Autodesk Inventor part; units mm, degrees
ref_plane "Work Plane1" through (-24, -152, 0) normal (0, -1, 0) x (1, 0, 0)
ref_plane "YZ Plane" through (0, 0, 0) normal (1, 0, 0) x (0, 1, 0)
ref_plane "XZ Plane" through (0, 0, 0) normal (0, 1, 0) x (-1, 0, 0)
sketch "Sketch1" plane through (0, 0, 0) normal (0, 0, 1) x (1, 0, 0)
  arc A0 (24, 0) -> (-24, 0) centre (0, 0) ccw
  line L0 (-24, 0) -> (-24, -152)
  line L1 (24, 0) -> (24, -152)
  dimension "d0" = 48
  dimension "d1" = 152
ref_plane "Work Plane1" through (-24, -152, 0) normal (0, -1, 0) x (1, 0, 0)
sketch "Sketch2" plane through (-24, -152, 0) normal (0, -1, 0) x (1, 0, 0)
  circle A0 centre (0, 0) radius 4
  point P0 (24, 0)
  dimension "d2" = 8
sweep "Колебание1" add profiles "Sketch2" path "Sketch1"
thread "Резьба1"
thread "Резьба2"
chamfer "Фаска1" distance 1 angle 45 2 edges at (28, -152, 0) (-28, -152, 0)
equation "\"d0\" = D + d_"
equation "\"d1\" = -d_ + H_ - 0.5 * D"
equation "\"d2\" = d_"
equation "\"d4\" = l_"
equation "\"d11\" = l_"
equation "\"D\" = 40"
equation "\"A_\" = 136"
equation "\"d_\" = 8"
equation "\"l_\" = 60"
properties part number "Скоба 40x170 ГОСТ 24137-80" material "Сталь, мягкая"
Part model, mm, in its own coordinate system. A direction names the side the tool comes from. Coordinates: 2 decimals unless noted, no trailing zeros. Order: outer loops, then holes, each group sorted by start corner. A loop starts at its lowest first (then second) coordinate and runs counter-clockwise, first axis right, second up.
(1) Pin check, flat tip, straight feed: pin 1 Ø1 at (y, z) = (-33, -1) entering from -X. Stop position of the tip, or through.
Check sheet entries:
pin 1: stops at x = -27.97
(2) Pull direction X, two halves, no side cores. Call faces 1 (the face through (24, -152, 0)), 2 (the face through (27.2, -74.4, -2.4)): pulls with the +X half, pulls with the -X half, needs draft (parallel to the pull), parting line crosses it, or undercut.
Check sheet entries:
face 1: needs draft
face 2: undercut
(3) Tool access for faces 3 (the face through (-24, -152, 0)), 4 (the face through (-27.2, -76.6, -2.4)): list every direction of +Z, -Z, +X, -X, +Y, -Y with a clear straight run to the whole face (end or side of a thin tool).
Check sheet entries:
face 3: +Z, -Z, +X, -X, -Y
face 4: -Y
(4) Slice it at A-A, the plane y = -5. Write the cut outline in (x, z).
Check sheet entries:
outline: circle Ø8 at (-24, 0); circle Ø8 at (24, 0)
(5) Slice it at B-B, the plane z = 0. Write the cut outline in (x, y), and give its area (3 significant figures).
Check sheet entries:
outline: (-28, -151) - (-27, -152) - (-21, -152) - (-20, -151) - (-20, 0) arc R20 cw to (20, 0) - (20, -151) - (21, -152) - (27, -152) - (28, -151) - (28, 0) arc R28 ccw to (-28, 0) - close
area: 3,030 mm2
(6) Probe L1, parallel to X at y = -76.5, z = -0.25; L2, parallel to X at y = -8, z = -3; L3, parallel to Y at x = 5, z = 2. List the from-to ranges inside material, lowest first.
Check sheet entries:
L1: x = -27.99 to -20.01, 20.01 to 27.99
L2: x = -26.65 to -21.35, 21.35 to 26.65
L3: y = 19.92 to 27.01
